from build123d import *

# Parameters (mm, degrees)
F1_DEPTH = 8
F2_W     = 4
F2_H     = 2.2
F3_DEPTH = 6
F4_R     = 0.8
F5_DEPTH = 5.101
F6_R     = 1


with BuildPart() as f1:
    # F0 (on Front) → F1 (new body)
    with BuildSketch(Plane.XZ):
        Polygon((-40, 4), (-40, 0), (0, 0), (40, 0), (40, 4), (0, 4), align=None)
    extrude(amount=F1_DEPTH)

    # F2 (on face) → F3 (join)
    with BuildSketch(Plane(origin=(0, 0, 0), x_dir=(1, 0, 0), z_dir=(0, 0, -1))):
        with Locations((-18.75, 4)):
            Rectangle(F2_W, F2_H)
        with Locations((18.75, 4)):
            Rectangle(F2_W, F2_H)
        with Locations((0, 4)):
            Rectangle(F2_W, F2_H)
    extrude(amount=F3_DEPTH)

    # F4 (on face) → F5 (cut, through all)
    with BuildSketch(Plane(origin=(0, -2.9, 0), x_dir=(-1, 0, 0), z_dir=(0, 1, 0))):
        with Locations((-18.75, -3.5)):
            Circle(F4_R)
        with Locations((18.75, -3.5)):
            Circle(F4_R)
        with Locations((0, -3.5)):
            Circle(F4_R)
    extrude(amount=-F5_DEPTH, mode=Mode.SUBTRACT)

    # F6
    f6_edges = [f1.edges().sort_by_distance(p)[0] for p in [
        (20.75, -4, -6),
        (16.75, -4, -6),
        (-16.75, -4, -6),
        (-20.75, -4, -6),
        (-2, -4, -6),
        (2, -4, -6),
    ]]
    fillet(f6_edges, radius=F6_R)


solid = f1.part
Can you work these out from the model? Positions are in its coordinate system, mm. A direction names the side the tool comes from. Give positions to 0.01 mm unless a question says otherwise; leave off trailing zeros. Loops run counter-clockwise (first coordinate to the right, second up) from the corner with the lowest first, then second, coordinate; pieces in that order, holes last. Notation, with made-up numbers: M 13,53.5 L 43,53.5 A26 ccw 43,82.5 Z; hole C 51.25,44 d4. An arc over 180 degrees is marked long. One line per item, written item: value. Start each with the question number.
1) I'm going to push flat-ended pins straight in: pin 1 (1.2 mm diameter, centred on x = -0.5, z = -1.5, fed in from +Y); pin 2 (1.1 mm diameter, centred on y = -4.5, z = -2, fed in from -X); pin 3 (4.5 mm diameter, centred on x = 1, z = -4.5, fed in from -Y). Where does each tip first touch, or does it pass through?
2) If we section it at C-C, the plane x = -10: Write out the boundary of the cut face in (y, z).
3) If we section it at A-A, the plane z = -2: Write out the boundary of the cut face in (x, y).
4) If we section it at D-D, the plane y = -1.5: Write out the boundary of the cut face in (x, z).
5) If we section it at B-B, the plane x = -18.75: Write out the boundary of the cut face in (y, z).
6) Thinking about a two-plate mould opening in X: for faces 1 (the face through (-1, 0, 2)), 2 (the face through (-40, -4, 2)), 3 (the face through (-2, -4, -2)), which applies, +X half, -X half, draft (parallel to the pull), parting line (faces both ways), or undercut?
7) On a 3-axis mill with a long thin cutter (end or side, diameter ignored), from which of +Z, -Z, +X, -X, +Y, -Y can I reach the whole of each face in a straight line? I mean faces 4 (the face through (20.75, -4, -2)), 5 (the face through (-19, -2.9, -2)), 6 (the face through (19, -5.1, -2)). Say none if no direction works.
8) If I drill on line 1 (X direction, y = -4.25, z = -2.25); line 2 (Z direction, x = 18.75, y = -4.6); line 3 (Z direction, x = 6.5, y = -6), over which ranges is the centre line in solid material (lowest first)? Write a range as [from, to].
Completed:
1. pin 1: stops at y = -2.9
1. pin 2: stops at x = -20.75
1. pin 3: stops at y = -5.1
2. outline: M -8,0 L 0,0 L 0,4 L -8,4 Z
3. outline: M -20.75,-5.1 L -16.75,-5.1 L -16.75,-2.9 L -20.75,-2.9 Z; M -2,-5.1 L 2,-5.1 L 2,-2.9 L -2,-2.9 Z; M 16.75,-5.1 L 20.75,-5.1 L 20.75,-2.9 L 16.75,-2.9 Z
4. outline: M -40,0 L 40,0 L 40,4 L -40,4 Z
5. outline: M -8,0 L -5.1,0 L -5.1,-2.7 L -2.9,-2.7 L -2.9,0 L 0,0 L 0,4 L -8,4 Z; M -5.1,-6 L -2.9,-6 L -2.9,-4.3 L -5.1,-4.3 Z
6. face 1: draft
6. face 2: -X half
6. face 3: undercut
7. face 4: -Z, +X, +Y, -Y
7. face 5: -Z, +X, -X, +Y
7. face 6: -Z, +X, -X, -Y
8. line 1: x = [-20.75, -16.75], [-2, 2], [16.75, 20.75]
8. line 2: z = [-6, -4.3], [-2.7, 4]
8. line 3: z = [0, 4]
